Input: part model. Units: mm. Frame: model coordinates. Give positions to 0.01 mm unless a question says otherwise; leave off trailing zeros. Loops run counter-clockwise (first coordinate to the right, second up) from the corner with the lowest first, then second, coordinate; pieces in that order, holes last. Notation, with made-up numbers: M -7,9.25 L 17,9.25 A3 ccw 17,13.25 Z; hole C 65.5,-35.5 d9. An arc over 180 degrees is marked long. Answer as a JSON object with one key per item and string values. Group by question number.
1) Section query B-B on x = 62. Return loops of the section in (y, z).
2) Ray query, L1, parallel to Y at x = 40, z = 1; L2, parallel to X at y = -2.5, z = 0.3; L3, parallel to Y at x = 73, z = 0.85. Return the intervals inside material, ascending.
3) Section query C-C on z = 0.25. Count the separate pieces of the cut face and the enclosed holes in it, plus the area to 3 significant figures.
4) Section query A-A on x = 49. Return loops of the section in (y, z), plus the area to 3 significant figures.
5) First-contact query: P1, Ø1.7, axis at x = 40, y = -25.83, coming from the -Z side; P2, Ø0.5, axis at x = 56.5, z = 0.5, coming from the +Y side. Flat tips, straight axial feed; report the tip coordinate or a pass-through.
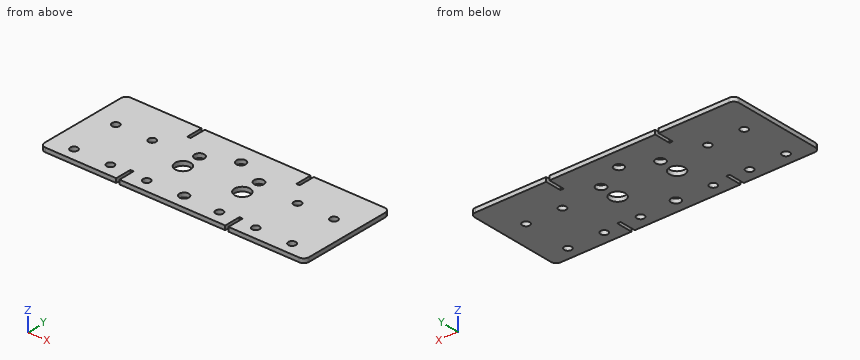
from build123d import *

# Parameters (mm, degrees)
SKETCH1_R           = 1.1303
SKETCH1_R_2         = 2.3495
SKETCH1_R_3         = 1.4732
SKETCH1_R_4         = 1.42
BOSS_EXTRUDE1_DEPTH = 1.27
FILLET1_R           = 1.5875


with BuildPart() as part:
    # Sketch1 → Boss-Extrude1 (new body)
    with BuildSketch(Plane.XY):
        Polygon((23, 0), (0, 0), (0, -30), (23, -30), (23, -25), (24, -25), (24, -30), (56, -30), (56, -25), (57, -25), (57, -30), (80, -30), (80, 0), (57, 0), (57, -5), (56, -5), (56, 0), (24, 0), (24, -5), (23, -5), align=None)
        with Locations((7, -26.225)):
            Circle(SKETCH1_R, mode=Mode.SUBTRACT)
        with Locations((18, -26.225)):
            Circle(SKETCH1_R, mode=Mode.SUBTRACT)
        with Locations((29, -26.225)):
            Circle(SKETCH1_R, mode=Mode.SUBTRACT)
        with Locations((31, -15.832468656)):
            Circle(SKETCH1_R_2, mode=Mode.SUBTRACT)
        with Locations((51, -26.225)):
            Circle(SKETCH1_R, mode=Mode.SUBTRACT)
        with Locations((62, -26.225)):
            Circle(SKETCH1_R, mode=Mode.SUBTRACT)
        with Locations((73, -26.225)):
            Circle(SKETCH1_R, mode=Mode.SUBTRACT)
        with Locations((49, -15.832468656)):
            Circle(SKETCH1_R_2, mode=Mode.SUBTRACT)
        with Locations((7, -11.525)):
            Circle(SKETCH1_R, mode=Mode.SUBTRACT)
        with Locations((18, -11.525)):
            Circle(SKETCH1_R, mode=Mode.SUBTRACT)
        with Locations((31, -10)):
            Circle(SKETCH1_R_3, mode=Mode.SUBTRACT)
        with Locations((49, -10)):
            Circle(SKETCH1_R_3, mode=Mode.SUBTRACT)
        with Locations((62, -11.525)):
            Circle(SKETCH1_R, mode=Mode.SUBTRACT)
        with Locations((73, -11.525)):
            Circle(SKETCH1_R, mode=Mode.SUBTRACT)
        with Locations((40, -5.832468656)):
            Circle(SKETCH1_R_4, mode=Mode.SUBTRACT)
        with Locations((40, -25.832468656)):
            Circle(SKETCH1_R_4, mode=Mode.SUBTRACT)
    extrude(amount=BOSS_EXTRUDE1_DEPTH)

    # Fillet1
    fillet1_edges = [part.edges().sort_by_distance(p)[0] for p in [
        (0, -30, 0.635),
        (0, 0, 0.635),
        (80, 0, 0.635),
        (80, -30, 0.635),
    ]]
    fillet(fillet1_edges, radius=FILLET1_R)


solid = part.part
Output:
{
 "1": {"outline": "M -30,0 L -27.36,0 L -27.36,1.27 L -30,1.27 Z; M -25.09,0 L -12.66,0 L -12.66,1.27 L -25.09,1.27 Z; M -10.39,0 L 0,0 L 0,1.27 L -10.39,1.27 Z"},
 "2": {"L1": "y = -30 to -27.25, -24.41 to -7.25, -4.41 to 0", "L2": "x = 0 to 23, 24 to 56, 57 to 80", "L3": "y = -30 to -27.36, -25.09 to -12.66, -10.39 to 0"},
 "3": {"separate pieces": "1", "enclosed holes": "16", "area": "2,280 mm^2"},
 "4": {"outline": "M -30,0 L -18.18,0 L -18.18,1.27 L -30,1.27 Z; M -13.48,0 L -11.47,0 L -11.47,1.27 L -13.48,1.27 Z; M -8.53,0 L 0,0 L 0,1.27 L -8.53,1.27 Z", "area": "28.4 mm^2"},
 "5": {"P1": "passes through", "P2": "stops at y = -5"}
}
